Here's how the part is built. I have some questions about the finished solid (model axes, mm). Face numbers are marked on the shaded views. A direction names the side the tool comes from. Round coordinates to 2 decimals unless told otherwise and drop trailing zeros. Order: outer loops, then holes, each group sorted by start corner. A loop starts at its lowest first (then second) coordinate and runs counter-clockwise, first axis right, second up. Notation, with made-up numbers: (50, 52.25) -> (66, 52.25) arc R10 cw to (66, 57.25) -> close; hole circle Ø7 at (-11.5, 2.5). An arc over 180 degrees is marked (long way). One line per item, written item: value.
```python
from build123d import *

# Parameters (mm, degrees)
BASE_DEPTH          = 2.5
BASE_DEPTH_BACK     = 2.5
SKETCH2_W           = 7.5
SKETCH2_H           = 15
SKETCH2_W_2         = 15
SKETCH2_H_2         = 7.5
BATTERYHOLDER_DEPTH = 25
SKETCH3_R           = 1.625
CUT_EXTRUDE1_DEPTH  = 10
SKETCH5_W           = 10
SKETCH5_H           = 13
BOSS_EXTRUDE2_DEPTH = 30
SKETCH6_R           = 3.625
CUT_EXTRUDE2_DEPTH  = 2.75
SKETCH7_R           = 3.625
CUT_EXTRUDE3_DEPTH  = 2.75
BOSS_EXTRUDE4_DEPTH = 25
CUT_EXTRUDE6_START  = -50
CUT_EXTRUDE6_DEPTH  = 63
CUT_EXTRUDE7_REACH  = 124.831
BOSS_EXTRUDE5_START = 2
BOSS_EXTRUDE5_DEPTH = 2
CUT_EXTRUDE8_REACH  = 126.183
SKETCH15_R          = 0.875
SKETCH16_W          = 6
SKETCH16_H          = 2.5
NUTCUT_DEPTH        = 10
SKETCH17_W          = 10
SKETCH17_H          = 15
BOSS_EXTRUDE6_DEPTH = 30
SKETCH18_R          = 4.125
CUT_EXTRUDE11_DEPTH = 2.75
CIRPATTERN2_COUNT   = 2


with BuildPart() as part:
    # Sketch1 → Base (new, two sides: drawn at the far end of the back side and taken through both)
    with BuildSketch(Plane(origin=(0, 0, 0), x_dir=(1, 0, 0), z_dir=(0, 1, 0)).offset(-BASE_DEPTH_BACK)):
        with BuildLine():
            Line((-50, 68.738635424), (-50, -68.738635424))
            ThreePointArc((-50, -68.738635424), (0, -85), (50, -68.738635424))
            Line((50, -68.738635424), (50, 68.738635424))
            ThreePointArc((50, 68.738635424), (0, 85), (-50, 68.738635424))
        make_face()
    extrude(amount=BASE_DEPTH + BASE_DEPTH_BACK)

    # Sketch2 → BatteryHolder (add)
    with BuildSketch(Plane(origin=(0, -2.5, 0), x_dir=(-1, 0, 0), z_dir=(0, -1, 0))):
        with Locations((45.25, 0)):
            Rectangle(SKETCH2_W, SKETCH2_H)
        with Locations((0, -39.75)):
            Rectangle(SKETCH2_W_2, SKETCH2_H_2)
        with Locations((-45.25, 0)):
            Rectangle(SKETCH2_W, SKETCH2_H)
        with Locations((0, 39.75)):
            Rectangle(SKETCH2_W_2, SKETCH2_H_2)
    extrude(amount=BATTERYHOLDER_DEPTH)

    # Sketch3 → Cut-Extrude1 (cut)
    with BuildSketch(Plane(origin=(0, -27.5, 0), x_dir=(-1, 0, 0), z_dir=(0, -1, 0))):
        with Locations(Location((45.5, 0, 0), (0, 0, 90))):
            Circle(SKETCH3_R)
        with Locations(Location((0, -40, 0), (0, 0, 90))):
            Circle(SKETCH3_R)
        with Locations(Location((-45.5, 0, 0), (0, 0, 90))):
            Circle(SKETCH3_R)
        with Locations(Location((0, 40, 0), (0, 0, 90))):
            Circle(SKETCH3_R)
    extrude(amount=-CUT_EXTRUDE1_DEPTH, mode=Mode.SUBTRACT)

    # Sketch5 → Boss-Extrude2 (add)
    with BuildSketch(Plane(origin=(0, -2.5, 0), x_dir=(-1, 0, 0), z_dir=(0, -1, 0))):
        with Locations((35, -42.5)):
            Rectangle(SKETCH5_W, SKETCH5_H)
        with Locations((-35, 42.5)):
            Rectangle(SKETCH5_W, SKETCH5_H)
    extrude(amount=BOSS_EXTRUDE2_DEPTH)

    # Sketch6 → Cut-Extrude2 (cut)
    with BuildSketch(Plane.ZY.offset(40)):
        with Locations((42.5, -25)):
            Circle(SKETCH6_R)
    extrude(amount=-CUT_EXTRUDE2_DEPTH, mode=Mode.SUBTRACT)

    # Sketch7 → Cut-Extrude3 (cut)
    with BuildSketch(Plane(origin=(40, 0, 0), x_dir=(0, 0, -1), z_dir=(1, 0, 0))):
        with Locations((42.5, -25)):
            Circle(SKETCH7_R)
    extrude(amount=-CUT_EXTRUDE3_DEPTH, mode=Mode.SUBTRACT)

    # Sketch12 → Boss-Extrude4 (add)
    with BuildSketch(Plane(origin=(0, -2.5, 0), x_dir=(-1, 0, 0), z_dir=(0, -1, 0))):
        Polygon((30, -49), (32.5, -49), (32.5, -68.5), (-17.5, -68.5), (-17.5, -36), (-7.5, -36), (-7.5, -43.5), (7.5, -43.5), (7.5, -36), (30, -36), align=None)
    boss_extrude4 = extrude(amount=BOSS_EXTRUDE4_DEPTH)

    # Sketch11 → Cut-Extrude6 (cut)
    with BuildSketch(Plane(origin=(0, 0, 0), x_dir=(0, 0, -1), z_dir=(1, 0, 0)).offset(CUT_EXTRUDE6_START)):
        with BuildLine():
            Line((-44.356601718, -14.393398282), (-44.356601718, 2.5))
            Line((-44.356601718, 2.5), (-61.856601718, 2.5))
            Line((-61.856601718, 2.5), (-61.856601718, -14.393398282))
            ThreePointArc((-61.856601718, -14.393398282), (-53.106601718, -23.143398282), (-44.356601718, -14.393398282))
        make_face()
    cut_extrude6 = extrude(amount=CUT_EXTRUDE6_DEPTH, mode=Mode.SUBTRACT)

    # Sketch13 → Cut-Extrude7 (cut, up to next)
    with BuildSketch(Plane.ZY.offset(32.5), mode=Mode.PRIVATE) as cut_extrude7_sk1:
        with BuildLine():
            Line((66.213203436, -14.393398282), (66.213203436, -2.5))
            Line((66.213203436, -2.5), (68.5, -2.5))
            Line((68.5, -2.5), (68.5, -27.5))
            Line((68.5, -27.5), (53.106601718, -27.5))
            ThreePointArc((53.106601718, -27.5), (62.374368671, -23.661165235), (66.213203436, -14.393398282))
        make_face()
    cut_extrude7_tool1 = extrude(cut_extrude7_sk1.sketch, amount=-CUT_EXTRUDE7_REACH, mode=Mode.PRIVATE) & part.part
    cut_extrude7 = cut_extrude7_tool1.solids().sort_by_distance((-32.5, -18.752717, 65.76063))[0]
    add(cut_extrude7, mode=Mode.SUBTRACT)

    # Sketch14 → Boss-Extrude5 (add)
    with BuildSketch(Plane.ZY.offset(32.5).offset(BOSS_EXTRUDE5_START)):
        with BuildLine():
            Line((49, -27.5), (49, -22.119867225))
            ThreePointArc((49, -22.119867225), (45.606759552, -18.900600018), (44.356601718, -14.393398282))
            Line((44.356601718, -14.393398282), (44.356601718, -11.393398282))
            Line((44.356601718, -11.393398282), (49.356601718, -11.393398282))
            Line((49.356601718, -11.393398282), (49.356601718, -14.393398282))
            ThreePointArc((49.356601718, -14.393398282), (53.106601718, -18.143398282), (56.856601718, -14.393398282))
            Line((56.856601718, -14.393398282), (56.856601718, -11.393398282))
            Line((56.856601718, -11.393398282), (66.213203436, -11.393398282))
            Line((66.213203436, -11.393398282), (66.213203436, -14.393398282))
            ThreePointArc((66.213203436, -14.393398282), (62.374368671, -23.661165235), (53.106601718, -27.5))
            Line((53.106601718, -27.5), (49, -27.5))
        make_face()
    boss_extrude5 = extrude(amount=-BOSS_EXTRUDE5_DEPTH)

    # Sketch15 → Cut-Extrude8 (cut, up to next)
    with BuildSketch(Plane.ZY.offset(34.5), mode=Mode.PRIVATE) as cut_extrude8_sk1:
        with Locations((58.606601718, -14.393398282)):
            Circle(SKETCH15_R)
    cut_extrude8_tool1 = extrude(cut_extrude8_sk1.sketch, amount=-CUT_EXTRUDE8_REACH, mode=Mode.PRIVATE) & part.part
    # Sketch15 → Cut-Extrude8 (cut, up to next)
    with BuildSketch(Plane.ZY.offset(34.5), mode=Mode.PRIVATE) as cut_extrude8_sk2:
        with Locations((47.606601718, -14.393398282)):
            Circle(SKETCH15_R)
    cut_extrude8_tool2 = extrude(cut_extrude8_sk2.sketch, amount=-CUT_EXTRUDE8_REACH, mode=Mode.PRIVATE) & part.part
    cut_extrude8_1 = cut_extrude8_tool1.solids().sort_by_distance((-34.5, -14.393398, 58.606602))[0]
    add(cut_extrude8_1, mode=Mode.SUBTRACT)
    cut_extrude8_2 = cut_extrude8_tool2.solids().sort_by_distance((-34.5, -14.393398, 47.606602))[0]
    add(cut_extrude8_2, mode=Mode.SUBTRACT)
    cut_extrude8 = cut_extrude8_1 + cut_extrude8_2  # Cut-Extrude8 as one shape, for the pattern or mirror that repeats it

    # Sketch16 → NutCut (cut)
    with BuildSketch(Plane(origin=(0, 0, 36), x_dir=(-1, 0, 0), z_dir=(0, 0, -1))):
        with Locations((0, -24.25)):
            Rectangle(SKETCH16_W, SKETCH16_H)
    extrude(amount=-NUTCUT_DEPTH, mode=Mode.SUBTRACT)

    # Sketch17 → Boss-Extrude6 (add)
    with BuildSketch(Plane(origin=(0, -2.5, 0), x_dir=(-1, 0, 0), z_dir=(0, -1, 0))):
        with Locations((-44, -42.5)):
            Rectangle(SKETCH17_W, SKETCH17_H)
    extrude(amount=BOSS_EXTRUDE6_DEPTH)

    # Sketch18 → Cut-Extrude11 (cut)
    with BuildSketch(Plane(origin=(49, 0, 0), x_dir=(0, 0, -1), z_dir=(1, 0, 0))):
        with Locations((-42.5, -25)):
            Circle(SKETCH18_R)
    extrude(amount=-CUT_EXTRUDE11_DEPTH, mode=Mode.SUBTRACT)

    # CirPattern2: Boss-Extrude4, Cut-Extrude6, Cut-Extrude7, Boss-Extrude5, Cut-Extrude8 ×2 about axis
    cirpattern2_axis = Axis((0, 0, 0), (0, 1, 0))
    add([boss_extrude4.rotate(cirpattern2_axis, i * 360 / CIRPATTERN2_COUNT) for i in range(1, CIRPATTERN2_COUNT)])
    add([cut_extrude6.rotate(cirpattern2_axis, i * 360 / CIRPATTERN2_COUNT) for i in range(1, CIRPATTERN2_COUNT)], mode=Mode.SUBTRACT)
    add([cut_extrude7.rotate(cirpattern2_axis, i * 360 / CIRPATTERN2_COUNT) for i in range(1, CIRPATTERN2_COUNT)], mode=Mode.SUBTRACT)
    add([boss_extrude5.rotate(cirpattern2_axis, i * 360 / CIRPATTERN2_COUNT) for i in range(1, CIRPATTERN2_COUNT)])
    add([cut_extrude8.rotate(cirpattern2_axis, i * 360 / CIRPATTERN2_COUNT) for i in range(1, CIRPATTERN2_COUNT)], mode=Mode.SUBTRACT)


solid = part.part
```
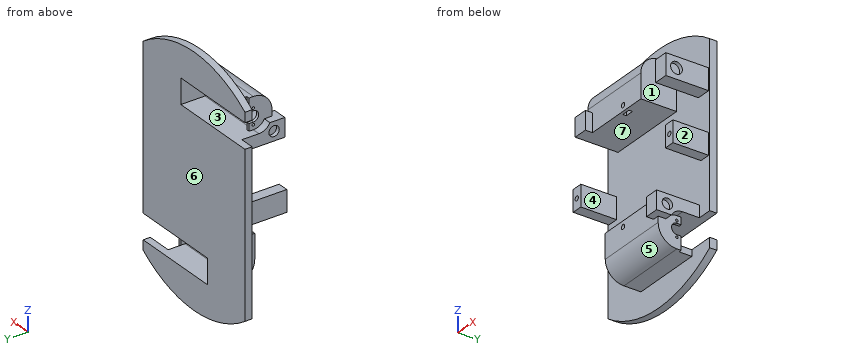
Q1. I want a section at A-A on y = -8.5. Write out the boundary of the cut face in (x, z), then the cut area to 3 significant figures.
Answers:
outline: (-49, -7.5) -> (-41.5, -7.5) -> (-41.5, 7.5) -> (-49, 7.5) -> close; (-40, 36) -> (17.5, 36) -> (17.5, 66.21) -> (-32.5, 66.21) -> (-32.5, 61.86) -> (13, 61.86) -> (13, 44.36) -> (-40, 44.36) -> close; (-17.5, -66.21) -> (32.5, -66.21) -> (32.5, -61.86) -> (-13, -61.86) -> (-13, -44.36) -> (40, -44.36) -> (40, -36) -> (-17.5, -36) -> close; (39, 35) -> (49, 35) -> (49, 50) -> (39, 50) -> close; (41.5, -7.5) -> (49, -7.5) -> (49, 7.5) -> (41.5, 7.5) -> close
area: 1,930 mm2
Q2. I want a section at D-D on x = -25. Write out the boundary of the cut face in (y, z), then the cut area to 3 significant figures.
Answers:
outline: (-27.5, 36) -> (-2.5, 36) -> (-2.5, -81.24) -> (2.5, -81.24) -> (2.5, 44.36) -> (-14.39, 44.36) arc R8.75 cw to (-14.39, 61.86) -> (2.5, 61.86) -> (2.5, 81.24) -> (-2.5, 81.24) -> (-2.5, 66.21) -> (-14.39, 66.21) arc R13.11 ccw to (-27.5, 53.11) -> close
area: 1,110 mm2
Q3. If we mould it in two halves opening along Z, with no side actions, what happens to the marked faces 5, 6 and 7? For each: pulls with the +Z half, pulls with the -Z half, needs draft (parallel to the pull), parting line crosses it, or undercut.
Answers:
face 5: pulls with the -Z half
face 6: needs draft
face 7: undercut
Q4. I want a section at B-B on x = -45.5. Write out the boundary of the cut face in (y, z) (3 decimals), then the cut area to 3 significant figures.
Answers:
outline: (-27.5, -7.5) -> (-2.5, -7.5) -> (-2.5, -71.797) -> (2.5, -71.797) -> (2.5, 44.357) -> (-2.5, 44.357) -> (-2.5, 7.5) -> (-27.5, 7.5) -> (-27.5, 1.625) -> (-17.5, 1.625) -> (-17.5, -1.625) -> (-27.5, -1.625) -> close; (-2.5, 61.857) -> (2.5, 61.857) -> (2.5, 71.797) -> (-2.5, 71.797) -> close
area: 973 mm2
Q5. I want a section at C-C on z = 29.5. Write out the boundary of the cut face in (x, y), then the cut area to 3 significant figures.
Answers:
outline: (-50, -2.5) -> (50, -2.5) -> (50, 2.5) -> (-50, 2.5) -> close
area: 500 mm2
Q6. I need wall thicknesses on line 1 along Z through (x, y) = (-4.5, -8); line 2 along X through (y, z) = (-14, 47.5); line 3 along Z through (x, y) = (39.5, -10). Which ranges of each line are inside material? Lowest first, please.
Answers:
line 1: -66.21 to -61.86, -44.36 to -36, 36 to 44.36, 61.86 to 66.21
line 2: 13 to 17.5, 39 to 49
line 3: -44.36 to -36, 35 to 50
Q7. Which directions (+Z, -Z, +X, -X, +Y, -Y) give clear straight access to the entire face, cutting with the end or side of a thin tool? Please do the marked faces 1, 2, 3 and 4.
Answers:
face 1: +Z, -Y
face 2: +Z, -Z, +X, -Y
face 3: +Y
face 4: +Z, -Z, -Y
Q8. For P1, Ø6, axis at x = 10.5, z = -45, coming from the +Y side; P2, Ø14.5, axis at y = -20.5, z = -40, coming from the +X side; P3, Ø1, axis at x = -34, y = -12.5, coming from the -Z side; P4, Ø8, axis at y = -22, z = -59, coming from the +X side, each with a flat end and sliding along its axis, tell me the tip position at first contact or that it passes through.
Answers:
P1: y = 2.5
P2: x = 40
P3: z = 36
P4: x = 34.5
